```python
from build123d import *
from build123d.topology import SkipClean

# Parameters (mm, degrees)
SKETCH1_R           = 50
BOSS_EXTRUDE1_DEPTH = 10
BOSS_EXTRUDE2_DEPTH = 10
BOSS_EXTRUDE3_START = 10
BOSS_EXTRUDE3_DEPTH = 10


with BuildPart() as part:
    # Sketch1 → Boss-Extrude1 (new body)
    with BuildSketch(Plane.XY):
        Circle(SKETCH1_R)
    extrude(amount=BOSS_EXTRUDE1_DEPTH)

    # Sketch2 → Boss-Extrude2 (add)
    with SkipClean():  # the faces are left unmerged after this step: merging them gives an invalid solid
        with BuildSketch(Plane.XY.offset(10)):
            with BuildLine():
                Line((-49.638694584, 6), (49.638694584, 6))
                ThreePointArc((49.638694584, 6), (50, 0), (49.638694584, -6))
                Line((49.638694584, -6), (-49.638694584, -6))
                ThreePointArc((-49.638694584, -6), (-50, 0), (-49.638694584, 6))
            make_face()
        extrude(amount=BOSS_EXTRUDE2_DEPTH)

    # Sketch3 → Boss-Extrude3 (add)
    with SkipClean():  # the faces are left unmerged after this step: merging them gives an invalid solid
        with BuildSketch(Plane(origin=(0, 0, 0), x_dir=(-1, 0, 0), z_dir=(0, 0, -1)).offset(BOSS_EXTRUDE3_START)):
            with BuildLine():
                Line((-5, 49.749371855), (-5, -49.749371855))
                ThreePointArc((-5, -49.749371855), (0, -50), (5, -49.749371855))
                Line((5, -49.749371855), (5, 49.749371855))
                ThreePointArc((5, 49.749371855), (0, 50), (-5, 49.749371855))
            make_face()
        extrude(amount=-BOSS_EXTRUDE3_DEPTH)


solid = part.part
```
Geometry: final body of the model. Coordinates: model frame, mm. A direction names the side the tool comes from. Round coordinates to 2 decimals unless told otherwise and drop trailing zeros. Write each loop counter-clockwise with the first axis right and the second up, starting at its lowest first coordinate (ties: lowest second). Pieces come first, ordered by that corner, then holes.
Item 1: Section query A-A (x = 37). Return loops of the section in (y, z), plus the area to 3 significant figures.
Item 2: Pin query (flat end, axial travel): P1, Ø11, axis at x = 1, z = 14.5, coming from the -Y side; P2, Ø11, axis at x = -13, z = 17.5, coming from the +Y side; P3, Ø5, axis at x = 11, y = -5, coming from the -Z side. Return the tip coordinate at first contact, or that it passes through.
Item 3: Material intervals for L1, parallel to Z at x = -26, y = 33; L2, parallel to Y at x = 1, z = 1.75; L3, parallel to X at y = 34.5, z = -6.75, sorted ascending.
Item 4: Section query D-D (z = -4.5). Return loops of the section in (x, y).
Item 5: Section query B-B (z = 12.75). Return loops of the section in (x, y), plus the area to 3 significant figures.
Item 6: Section query C-C (y = -43). Return loops of the section in (x, z).
Item 7: Set-up query: faces 1 (the face through (-1, 6, 15)), 2 (the face through (1, 0, 20)), 3 (the face through (-5, -1, -5)), 4 (the face through (5, 1, -5)), 5 (the face through (1, -6, 15)). Return all of +Z, -Z, +X, -X, +Y, -Y with unobstructed straight access to the full face (end or side cutting, diameter ignored); none if empty.
Completed:
1. outline: (-33.63, 0) - (33.63, 0) - (33.63, 10) - (6, 10) - (6, 20) - (-6, 20) - (-6, 10) - (-33.63, 10) - close
1. area: 793 mm2
2. P1: stops at y = -50
2. P2: stops at y = 6
2. P3: stops at z = 0
3. L1: z = 0 to 10
3. L2: y = -49.99 to 49.99
3. L3: x = -5 to 5
4. outline: (-5, -49.75) arc R50 ccw to (5, -49.75) - (5, 49.75) arc R50 ccw to (-5, 49.75) - close
5. outline: (-49.64, -6) - (49.64, -6) arc R50 ccw to (49.64, 6) - (-49.64, 6) arc R50 ccw to start
5. area: 1,200 mm2
6. outline: (-25.51, 0) - (-5, 0) - (-5, -10) - (5, -10) - (5, 0) - (25.51, 0) - (25.51, 10) - (-25.51, 10) - close
7. face 1: +Z, +X, -X, +Y
7. face 2: +Z, +X, -X, +Y, -Y
7. face 3: -Z, -X, +Y, -Y
7. face 4: -Z, +X, +Y, -Y
7. face 5: +Z, +X, -X, -Y
